Design review of the part built by this model. Coordinates are the model's own, in mm. Coordinates: 2 decimals unless noted, no trailing zeros. Write each loop counter-clockwise with the first axis right and the second up, starting at its lowest first coordinate (ties: lowest second). Pieces come first, ordered by that corner, then holes. Notation, with made-up numbers: (19.25, 24.5) - (28.25, 24.5) arc R23 cw to (28.25, 33.5) - close; hole circle Ø9 at (40, 23.5). An arc over 180 degrees is marked (long way). Use a Markdown table: item, result.
from build123d import *

# Parameters (mm, degrees)
SKETCH1_R           = 9.5
SKETCH1_W           = 40
SKETCH1_H           = 6
BOSS_EXTRUDE1_DEPTH = 6


with BuildPart() as part:
    # Sketch1 → Boss-Extrude1 (new body)
    with BuildSketch(Plane.XY):
        with BuildLine():
            Line((-35.529687849, 42.131147541), (314.470312151, 42.131147541))
            ThreePointArc((314.470312151, 42.131147541), (354.470312151, 2.131147541), (314.470312151, -37.868852459))
            Line((314.470312151, -37.868852459), (-35.529687849, -37.868852459))
            ThreePointArc((-35.529687849, -37.868852459), (-75.529687849, 2.131147541), (-35.529687849, 42.131147541))
        make_face()
        with Locations((-35.529687849, 2.131147541)):
            Circle(SKETCH1_R, mode=Mode.SUBTRACT)
        with Locations((314.470312151, 2.131147541)):
            Circle(SKETCH1_R, mode=Mode.SUBTRACT)
        with Locations((139.470312151, 19.131147541)):
            Rectangle(SKETCH1_W, SKETCH1_H, mode=Mode.SUBTRACT)
        with Locations((244.470312151, 19.131147541)):
            Rectangle(SKETCH1_W, SKETCH1_H, mode=Mode.SUBTRACT)
        with Locations((34.470312151, 19.131147541)):
            Rectangle(SKETCH1_W, SKETCH1_H, mode=Mode.SUBTRACT)
    extrude(amount=BOSS_EXTRUDE1_DEPTH)


solid = part.part
(1) Take a section at C-C on z = 1.9. Write out the cut boundary in (x, y).
Determined:
| item | result |
|---|---|
| outline | (-35.53, -37.87) - (314.47, -37.87) arc R40 ccw to (314.47, 42.13) - (-35.53, 42.13) arc R40 ccw to start; hole circle Ø19 at (-35.53, 2.13); hole (14.47, 16.13) - (54.47, 16.13) - (54.47, 22.13) - (14.47, 22.13) - close; hole (119.47, 16.13) - (159.47, 16.13) - (159.47, 22.13) - (119.47, 22.13) - close; hole (224.47, 16.13) - (264.47, 16.13) - (264.47, 22.13) - (224.47, 22.13) - close; hole circle Ø19 at (314.47, 2.13) |
(2) Take a section at B-B on y = 8. Write out the cut boundary in (x, z).
Determined:
| item | result |
|---|---|
| outline | (-75.1, 0) - (-43, 0) - (-43, 6) - (-75.1, 6) - close; (-28.06, 0) - (307, 0) - (307, 6) - (-28.06, 6) - close; (321.94, 0) - (354.04, 0) - (354.04, 6) - (321.94, 6) - close |
(3) Take a section at D-D on y = -33. Write out the cut boundary in (x, z), and give its area (3 significant figures).
Determined:
| item | result |
|---|---|
| outline | (-54.66, 0) - (333.6, 0) - (333.6, 6) - (-54.66, 6) - close |
| area | 2,330 mm2 |
(4) Draft analysis for pull direction X (two halves, no side actions). For faces 1 (the cylindrical face through (354.46, 3.01, 2.96)), 2 (the cylindrical face through (323.246, -1.507, 2.958)), 3 (the flat face through (142, 3, 0)), state which applies: +X half, -X half, draft (parallel to the pull), parting line (faces both ways), or undercut.
Determined:
| item | result |
|---|---|
| face 1 | +X half |
| face 2 | undercut |
| face 3 | draft |
(5) Take a section at A-A on x = 140. Write out the cut boundary in (y, z).
Determined:
| item | result |
|---|---|
| outline | (-37.87, 0) - (16.13, 0) - (16.13, 6) - (-37.87, 6) - close; (22.13, 0) - (42.13, 0) - (42.13, 6) - (22.13, 6) - close |
(6) For L1, parallel to X at y = 3, z = 4.65; L2, parallel to Y at x = 147.5, z = 5.25; L3, parallel to X at y = 6, z = 5.7, list the stretches that pass through material, from the lowest coordinate up. Write a range as from..to.
Determined:
| item | result |
|---|---|
| L1 | -75.52..-44.99, -26.07..305.01, 323.93..354.46 |
| L2 | -37.87..16.13, 22.13..42.13 |
| L3 | -75.34..-44.21, -26.85..305.79, 323.15..354.28 |
(7) For pin 1 (1.8 mm diameter, centred on y = 20.5, z = 2, fed in from +X); pin 2 (2 mm diameter, centred on y = -15, z = 2, fed in from -X); pin 3 (15 mm diameter, centred on x = 314.47, y = 2.13, fed in from +Z); pin 4 (1.8 mm diameter, centred on y = 20.5, z = 1.5, fed in from -X), all flat-tipped, find the tip position at first contact; note any pin that passes through.
Determined:
| item | result |
|---|---|
| pin 1 | x = 350.45 |
| pin 2 | x = -72.13 |
| pin 3 | through |
| pin 4 | x = -71.51 |
